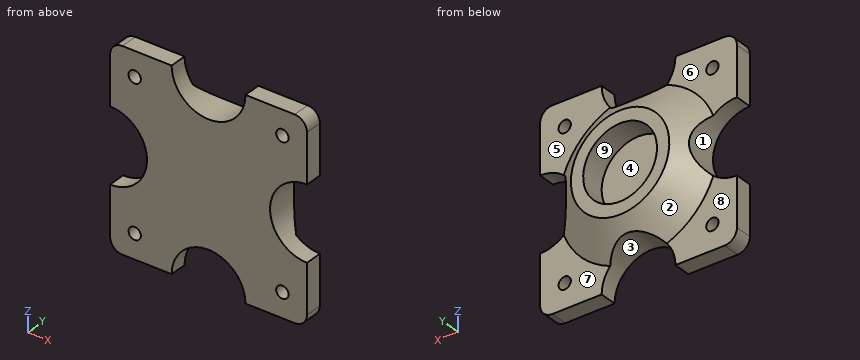
from build123d import *

# Parameters (mm, degrees)
BOSS_EXTRUDE1_DEPTH = 8.89
SKETCH3_R           = 19.05
SKETCH3_R_2         = 3.175
CUT_EXTRUDE1_DEPTH  = 76.016052282
SKETCH3_3_R         = 19.05
CUT_EXTRUDE2_DEPTH  = 12.7


with BuildPart() as part:
    # Sketch1 → Boss-Extrude1 (new body)
    with BuildSketch(Plane(origin=(0, 0, 0), x_dir=(1, 0, 0), z_dir=(0, 1, 0))):
        with BuildLine():
            Line((-44.45, -50.8), (44.45, -50.8))
            ThreePointArc((44.45, -50.8), (48.940128061, -48.940128061), (50.8, -44.45))
            Line((50.8, -44.45), (50.8, 44.45))
            ThreePointArc((50.8, 44.45), (48.940128061, 48.940128061), (44.45, 50.8))
            Line((44.45, 50.8), (-44.45, 50.8))
            ThreePointArc((-44.45, 50.8), (-48.940128061, 48.940128061), (-50.8, 44.45))
            Line((-50.8, 44.45), (-50.8, -44.45))
            ThreePointArc((-50.8, -44.45), (-48.940128061, -48.940128061), (-44.45, -50.8))
        make_face()
    extrude(amount=BOSS_EXTRUDE1_DEPTH)

    # Sketch2 → Revolve1 (revolve)
    with BuildSketch(Plane.XY, mode=Mode.PRIVATE) as revolve1_sk:
        Polygon((0, 21.59), (0, 8.89), (41.275, 8.89), (25.4, 21.59), align=None)
    revolve(revolve1_sk.sketch.rotate(Axis((0, -26.658191996, 0), (0, 1, 0)), 90), axis=Axis((0, -26.658191996, 0), (0, 1, 0)))

    # Sketch3 → Cut-Extrude1 (cut, through all)
    with BuildSketch(Plane(origin=(0, 21.59, 0), x_dir=(1, 0, 0), z_dir=(0, 1, 0))):
        with Locations((-50.8, 0)):
            Circle(SKETCH3_R)
        with Locations((0, 50.8)):
            Circle(SKETCH3_R)
        with Locations((0, -50.8)):
            Circle(SKETCH3_R)
        with Locations((50.8, 0)):
            Circle(SKETCH3_R)
        with Locations(Location((38.1, -38.1, 0), (0, 0, 270))):
            Circle(SKETCH3_R_2)
        with Locations(Location((38.1, 38.1, 0), (0, 0, 270))):
            Circle(SKETCH3_R_2)
        with Locations(Location((-38.1, 38.1, 0), (0, 0, 270))):
            Circle(SKETCH3_R_2)
        with Locations(Location((-38.1, -38.1, 0), (0, 0, 270))):
            Circle(SKETCH3_R_2)
    extrude(amount=-CUT_EXTRUDE1_DEPTH, mode=Mode.SUBTRACT)

    # Sketch3<3> → Cut-Extrude2 (cut)
    with BuildSketch(Plane(origin=(0, 21.59, 0), x_dir=(1, 0, 0), z_dir=(0, 1, 0))):
        with Locations(Location((0, 0, 0), (0, 0, 270))):
            Circle(SKETCH3_3_R)
    extrude(amount=-CUT_EXTRUDE2_DEPTH, mode=Mode.SUBTRACT)


solid = part.part
Part model, mm, in its own coordinate system. Face numbers are marked on the shaded views. A direction names the side the tool comes from. Round coordinates to 2 decimals unless told otherwise and drop trailing zeros. Write each loop counter-clockwise with the first axis right and the second up, starting at its lowest first coordinate (ties: lowest second). Pieces come first, ordered by that corner, then holes. Notation, with made-up numbers: (-24.75, -11) - (11.25, -11) arc R20 cw to (11.25, -4) - close; hole circle Ø9 at (11.5, -8). An arc over 180 degrees is marked (long way). Use CSV: the item, a comma, the result in double quotes.
Item 1: Tool access for the marked faces 5, 6, 7, 8 and 9: list every direction of +Z, -Z, +X, -X, +Y, -Y with a clear straight run to the whole face (end or side of a thin tool).
Results list:
face 5,"+Z, +X, +Y"
face 6,"+Z, -X, +Y"
face 7,"-Z, +X, +Y"
face 8,"-Z, -X, +Y"
face 9,"+Y"
Item 2: Slice it at B-B, the plane x = 0. Write the cut outline in (y, z), then the cut area to 3 significant figures.
Results list:
outline,"(0, -31.75) - (16.51, -31.75) - (21.59, -25.4) - (21.59, -19.05) - (8.89, -19.05) - (8.89, 19.05) - (21.59, 19.05) - (21.59, 25.4) - (16.51, 31.75) - (0, 31.75) - close"
area,"855 mm²"
Item 3: Flat gauge pins, fed straight in: P1, Ø1, axis at x = 20.5, z = -38.5, coming from the +Y side; P2, Ø3, axis at x = -20, z = 23.5, coming from the +Y side; P3, Ø8, axis at y = 18, z = -18.5, coming from the +X side. Where does each tip first touch, or does it go through?
Results list:
P1,"stops at y = 8.89"
P2,"stops at y = 18.42"
P3,"stops at x = 30.05"
Item 4: Wall check: L1, parallel to X at y = 1.5, z = -40.5; L2, parallel to X at y = 2, z = -38.1 (3 decimals); L3, parallel to Y at x = 29.5, z = 39.5. Give the ranges that are in metal, low to high.
Results list:
L1,"x = -50.8 to -40.18, -36.02 to -16.03, 16.03 to 36.02, 40.18 to 50.8"
L2,"x = -50.8 to -41.275, -34.925 to -14.199, 14.199 to 34.925, 41.275 to 50.8"
L3,"y = 0 to 8.89"
Item 5: Slice it at C-C, the plane z = 0. Write the cut outline in (x, y), then the cut area to 3 significant figures.
Results list:
outline,"(-31.75, 0) - (31.75, 0) - (31.75, 16.51) - (25.4, 21.59) - (19.05, 21.59) - (19.05, 8.89) - (-19.05, 8.89) - (-19.05, 21.59) - (-25.4, 21.59) - (-31.75, 16.51) - close"
area,"855 mm²"
Item 6: Pull direction X, two halves, no side cores. Call the marked faces 1, 2, 3 and 4: pulls with the +X half, pulls with the -X half, needs draft (parallel to the pull), parting line crosses it, or undercut.
Results list:
face 1,"pulls with the -X half"
face 2,"parting line crosses it"
face 3,"undercut"
face 4,"undercut"
Item 7: Slice it at A-A, the plane z = 43. Write the cut outline in (x, y).
Results list:
outline,"(-50.8, 0) - (-17.38, 0) - (-17.38, 8.89) - (-50.8, 8.89) - close; (17.38, 0) - (50.8, 0) - (50.8, 8.89) - (17.38, 8.89) - close"
